Answer from the drawing. Dimensions are ordinates in mm from the lowest x, y and z of the part. Give positions to 0.01 mm unless a question says otherwise; leave off trailing zeros. Order: outer loops, then holes, each group sorted by start corner. A loop starts at its lowest first (then second) coordinate and runs counter-clockwise, first axis right, second up. Notation, with made-up numbers: (79.5, 10.5) - (88.5, 10.5) arc R19 cw to (88.5, 19.5) - close; hole circle Ø1 at (32.5, 86.5). An arc over 180 degrees is marked (long way). Use a Markdown table: item, result. Add a question column.
1) Flat-ended cylindrical pins translate along their axes: pin 1 (2 mm diameter, centred on x = 6, y = 5.5, fed in from +Z); pin 2 (6 mm diameter, centred on x = 7.5, z = 3.5, fed in from -Y); pin 3 (1 mm diameter, centred on x = 5, z = 8, fed in from +Y); pin 4 (6 mm diameter, centred on x = 5.5, z = 7, fed in from -Y). Find the tip coordinate at first contact, or state that the pin passes through.
2) Find section B-B, the plane z = 4.5. Determine the outline of the cut face in (x, y).
3) The mould has two halves that part along X. Classify the marked faces 1, 2 and 3: released by +X, released by -X, zero draft, split by the parting line, or undercut.
4) Find section A-A, the plane x = 5. Determine the outline of the cut face in (y, z) (1 decimal).
5) Straight lines are drawn through the part: line 1 (Y direction, x = 5, z = 7.5); line 2 (Z direction, x = 5.5, y = 6); line 3 (Y direction, x = 4.25, z = 2.75). For each, find the intervals that lie inside material, in ascending order.
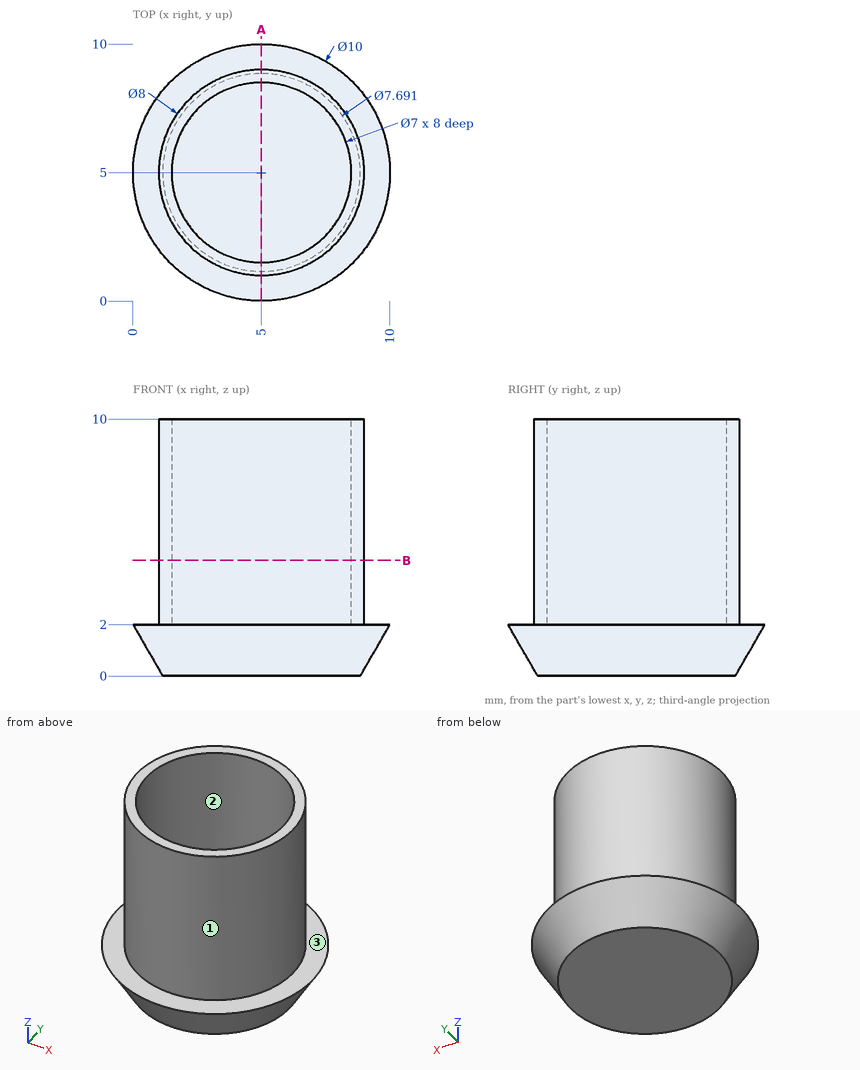
The answers:
| question | item | result |
|---|---|---|
| 1 | pin 1 | z = 2 |
| 1 | pin 2 | y = 0 |
| 1 | pin 3 | y = 9 |
| 1 | pin 4 | y = 1 |
| 2 | outline | circle Ø8 at (5, 5); hole circle Ø7 at (5, 5) |
| 3 | face 1 | split by the parting line |
| 3 | face 2 | undercut |
| 3 | face 3 | zero draft |
| 4 | outline | (0, 2) - (1.2, 0) - (8.8, 0) - (10, 2) - (9, 2) - (9, 10) - (8.5, 10) - (8.5, 2) - (1.5, 2) - (1.5, 10) - (1, 10) - (1, 2) - close |
| 5 | line 1 | 1 to 1.5, 8.5 to 9 |
| 5 | line 2 | 0 to 2 |
| 5 | line 3 | 1.07 to 1.58, 8.42 to 8.93 |
